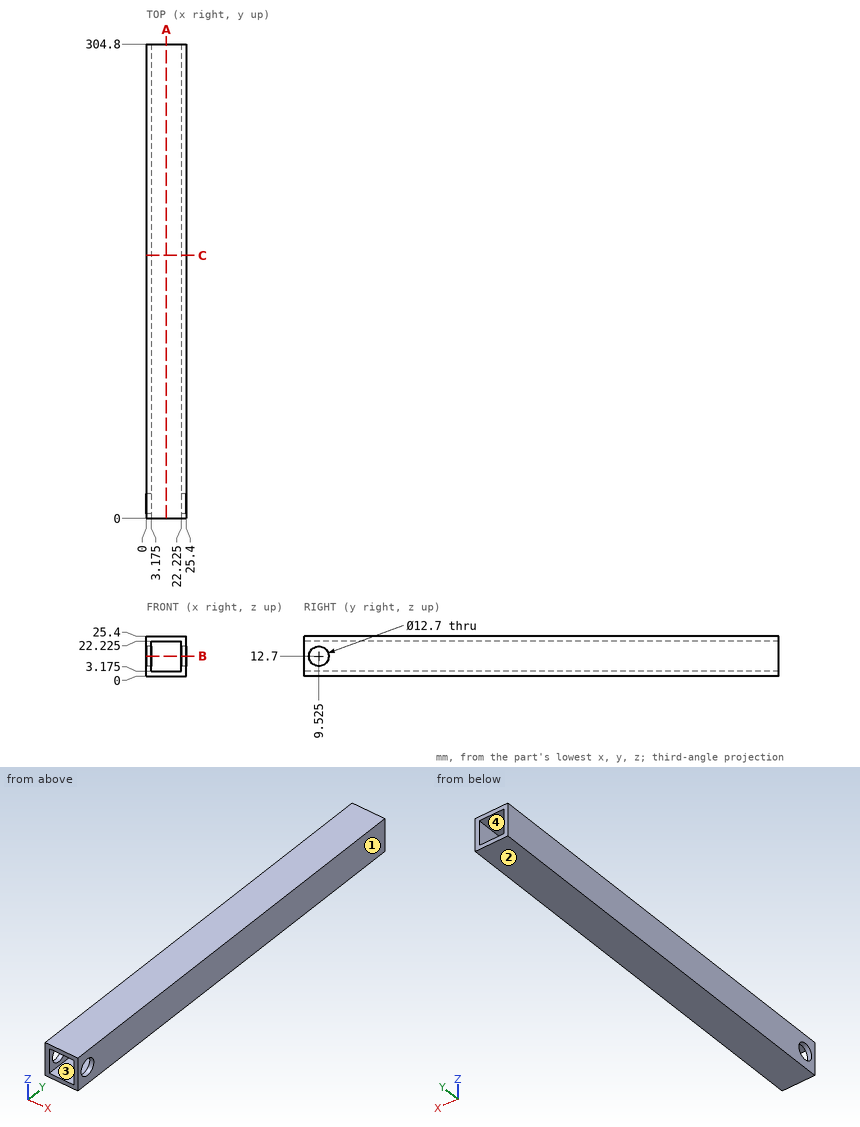
Here's the drawing with two shaded views (mm, measured from the low corner). I have some questions. Give positions to 0.01 mm unless a question says otherwise; leave off trailing zeros. Loops run counter-clockwise (first coordinate to the right, second up) from the corner with the lowest first, then second, coordinate; pieces in that order, holes last. Notation, with made-up numbers: (42, 80.5) - (84, 80.5) arc R23 ccw to (84, 118.5) - close; hole circle Ø5 at (-0.75, 20). An arc over 180 degrees is marked (long way). Answer in a Markdown table with one row per item. Add a question column.
Q1. If we section it at A-A (x = 12.75): List the corners of the cut face in (y, z) for me (3 decimals), plus the area to 3 significant figures.
Q2. We'd pull the mould along X, two halves only. Please class the marked faces 1, 2, 3 and 4: +X half, -X half, draft (parallel to the pull), parting line (faces both ways), or undercut.
Q3. If we section it at B-B (z = 12.7): List the corners of the cut face in (x, y) for me (3 decimals), plus the area to 3 significant figures.
Q4. Please list where this line runs through material, in increasing order: L1, parallel to Z at x = 8.75, y = 116.5 (3 decimals). Write a range as from..to.
Q5. If we section it at C-C (y = 169): List the corners of the cut face in (x, z) for me (3 decimals).
The answers:
| question | item | result |
|---|---|---|
| 1 | outline | (0, 0) - (304.8, 0) - (304.8, 3.175) - (0, 3.175) - close; (0, 22.225) - (304.8, 22.225) - (304.8, 25.4) - (0, 25.4) - close |
| 1 | area | 1,940 mm^2 |
| 2 | face 1 | +X half |
| 2 | face 2 | draft |
| 2 | face 3 | undercut |
| 2 | face 4 | undercut |
| 3 | outline | (0, 0) - (3.175, 0) - (3.175, 3.175) - (0, 3.175) - close; (0, 15.875) - (3.175, 15.875) - (3.175, 304.8) - (0, 304.8) - close; (22.225, 0) - (25.4, 0) - (25.4, 3.175) - (22.225, 3.175) - close; (22.225, 15.875) - (25.4, 15.875) - (25.4, 304.8) - (22.225, 304.8) - close |
| 3 | area | 1,850 mm^2 |
| 4 | L1 | z = 0..3.175, 22.225..25.4 |
| 5 | outline | (0, 0) - (25.4, 0) - (25.4, 25.4) - (0, 25.4) - close; hole (3.175, 3.175) - (22.225, 3.175) - (22.225, 22.225) - (3.175, 22.225) - close |
